Here's the drawing with two shaded views (mm, measured from the low corner). I have some questions. A direction names the side the tool comes from. Round coordinates to 2 decimals unless told otherwise and drop trailing zeros. Loops run counter-clockwise (first coordinate to the right, second up) from the corner with the lowest first, then second, coordinate; pieces in that order, holes last. Notation, with made-up numbers: (72.5, 23) -> (79.5, 23) arc R36 ccw to (79.5, 62) -> close; hole circle Ø2 at (19, 26.25). An arc over 180 degrees is marked (long way). Use a Markdown table: item, result.
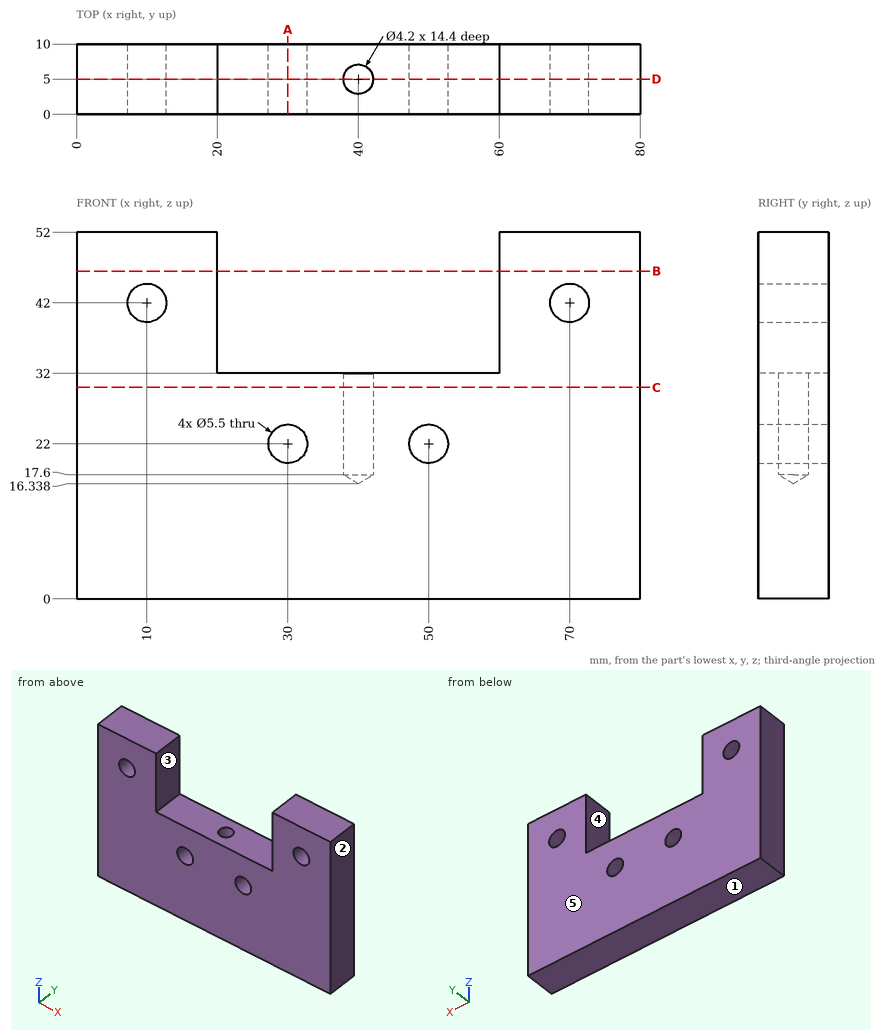
1. I want a section at B-B (z = 46.5). Please give me the cut outline in (x, y).
Answer sheet:
| item | result |
|---|---|
| outline | (0, 0) -> (20, 0) -> (20, 10) -> (0, 10) -> close; (60, 0) -> (80, 0) -> (80, 10) -> (60, 10) -> close |
2. I need wall thicknesses on line 1 (X direction, y = 3.75, z = 50); line 2 (Z direction, x = 30, y = 4.75); line 3 (Z direction, x = 10, y = 7.5). Which ranges of each line are inside material? Lowest first, please.
Answer sheet:
| item | result |
|---|---|
| line 1 | x = 0 to 20, 60 to 80 |
| line 2 | z = 0 to 19.25, 24.75 to 32 |
| line 3 | z = 0 to 39.25, 44.75 to 52 |
3. Will this pin go through, and if not, where does the flat tip stop? pin 1 Ø3 at (x, y) = (50.5, 9) entering from +Z.
Answer sheet:
| item | result |
|---|---|
| pin 1 | stops at z = 32 |
4. I want a section at C-C (z = 30). Please give me the cut outline in (x, y).
Answer sheet:
| item | result |
|---|---|
| outline | (0, 0) -> (80, 0) -> (80, 10) -> (0, 10) -> close; hole circle Ø4.2 at (40, 5) |
5. I want a section at D-D (y = 5). State how many separate pieces and enclosed holes the cut face has, plus the area to 3 significant figures.
Answer sheet:
| item | result |
|---|---|
| separate pieces | 1 |
| enclosed holes | 4 |
| area | 3,200 mm² |
6. I want a section at A-A (x = 30). Please give me the cut outline in (y, z), plus the area to 3 significant figures.
Answer sheet:
| item | result |
|---|---|
| outline | (0, 0) -> (10, 0) -> (10, 19.25) -> (0, 19.25) -> close; (0, 24.75) -> (10, 24.75) -> (10, 32) -> (0, 32) -> close |
| area | 265 mm² |
7. Which directions (+Z, -Z, +X, -X, +Y, -Y) give clear straight access to the entire face, cutting with the end or side of a thin tool? Please do the marked faces 4 and 5.
Answer sheet:
| item | result |
|---|---|
| face 4 | +Z, +Y, -Y |
| face 5 | +Z, -Z, +X, -X, +Y |
8. If we mould it in two halves opening along X, with no side actions, what happens to the marked faces 1, 2 and 3? For each: +X half, -X half, draft (parallel to the pull), parting line (faces both ways), or undercut.
Answer sheet:
| item | result |
|---|---|
| face 1 | draft |
| face 2 | +X half |
| face 3 | undercut |
